from build123d import *
from build123d import SkipClean  # not in build123d's __all__

# Parameters (mm, degrees)
F0_W     = 71.95
F0_H     = 24.75
F1_DEPTH = 2
F2_DEPTH = 5


with BuildPart() as f1:
    # F0 (on Top) → F1 (new body)
    with BuildSketch(Plane.XY):
        with BuildLine():
            Line((34.5, 15), (-34.5, 15))
            ThreePointArc((-34.5, 15), (-36.6339745962, 12.1277186767), (-40, 13.3416876048))
            Line((-40, 13.3416876048), (-40, -14.8416876048))
            ThreePointArc((-40, -14.8416876048), (-37.4068848056, -13.5014454214), (-34.9019237886, -15))
            Line((-34.9019237886, -15), (34.9019237886, -15))
            ThreePointArc((34.9019237886, -15), (37.4068848056, -13.5014454214), (40, -14.8416876048))
            Line((40, -14.8416876048), (40, 13.3416876048))
            ThreePointArc((40, 13.3416876048), (36.6339745962, 12.1277186767), (34.5, 15))
        make_face()
        Rectangle(F0_W, F0_H, mode=Mode.SUBTRACT)
        with BuildLine():
            Line((-34.5, 15), (-36, 15))
            ThreePointArc((-36, 15), (-37.5, 13.5), (-39, 15))
            Line((-39, 15), (-40, 15))
            Line((-40, 15), (-40, 13.3416876048))
            ThreePointArc((-40, 13.3416876048), (-36.6339745962, 12.1277186767), (-34.5, 15))
        make_face()
        with BuildLine():
            Line((36, 15), (34.5, 15))
            ThreePointArc((34.5, 15), (36.6339745962, 12.1277186767), (40, 13.3416876048))
            Line((40, 13.3416876048), (40, 15))
            Line((40, 15), (39, 15))
            ThreePointArc((39, 15), (37.5, 13.5), (36, 15))
        make_face()
        with BuildLine():
            Line((40, -15), (40, -14.8416876048))
            ThreePointArc((40, -14.8416876048), (37.4068848056, -13.5014454214), (34.9019237886, -15))
            Line((34.9019237886, -15), (37.5, -15))
            Line((37.5, -15), (40, -15))
        make_face()
        with BuildLine():
            ThreePointArc((-34.9019237886, -15), (-37.4068848056, -13.5014454214), (-40, -14.8416876048))
            Line((-40, -14.8416876048), (-40, -15))
            Line((-40, -15), (-37.5, -15))
            Line((-37.5, -15), (-34.9019237886, -15))
        make_face()
    extrude(amount=F1_DEPTH)

    # F0 (on Top) → F2 (join)
    with BuildSketch(Plane.XY):
        with BuildLine():
            Line((-34.5, 15), (-36, 15))
            ThreePointArc((-36, 15), (-37.5, 13.5), (-39, 15))
            Line((-39, 15), (-40, 15))
            Line((-40, 15), (-40, 13.3416876048))
            ThreePointArc((-40, 13.3416876048), (-36.6339745962, 12.1277186767), (-34.5, 15))
        make_face()
        with BuildLine():
            ThreePointArc((-39, 15), (-37.5, 16.5), (-36, 15))
            Line((-36, 15), (-34.5, 15))
            ThreePointArc((-34.5, 15), (-38.3660254038, 17.8722813233), (-40, 13.3416876048))
            Line((-40, 13.3416876048), (-40, 15))
            Line((-40, 15), (-39, 15))
        make_face()
        with BuildLine():
            Line((-40, -15), (-40, -14.8416876048))
            ThreePointArc((-40, -14.8416876048), (-38.3660254038, -19.3722813233), (-34.5, -16.5))
            ThreePointArc((-34.5, -16.5), (-34.6022225211, -15.7235428647), (-34.9019237886, -15))
            Line((-34.9019237886, -15), (-37.5, -15))
            Line((-37.5, -15), (-40, -15))
        make_face()
        with BuildLine():
            ThreePointArc((-36, -16.5), (-38.5606601718, -17.5606601718), (-37.5, -15))
            ThreePointArc((-37.5, -15), (-36.4393398282, -15.4393398282), (-36, -16.5))
        make_face(mode=Mode.SUBTRACT)
        with BuildLine():
            ThreePointArc((-34.9019237886, -15), (-37.4068848056, -13.5014454214), (-40, -14.8416876048))
            Line((-40, -14.8416876048), (-40, -15))
            Line((-40, -15), (-37.5, -15))
            Line((-37.5, -15), (-34.9019237886, -15))
        make_face()
        with BuildLine():
            ThreePointArc((40.5, -16.5), (40.3722813233, -15.6339745962), (40, -14.8416876048))
            Line((40, -14.8416876048), (40, -15))
            Line((40, -15), (37.5, -15))
            Line((37.5, -15), (34.9019237886, -15))
            ThreePointArc((34.9019237886, -15), (36.7235428647, -19.3977774789), (40.5, -16.5))
        make_face()
        with BuildLine():
            ThreePointArc((39, -16.5), (36.4393398282, -17.5606601718), (37.5, -15))
            ThreePointArc((37.5, -15), (38.5606601718, -15.4393398282), (39, -16.5))
        make_face(mode=Mode.SUBTRACT)
        with BuildLine():
            Line((40, -15), (40, -14.8416876048))
            ThreePointArc((40, -14.8416876048), (37.4068848056, -13.5014454214), (34.9019237886, -15))
            Line((34.9019237886, -15), (37.5, -15))
            Line((37.5, -15), (40, -15))
        make_face()
        with BuildLine():
            ThreePointArc((40.5, 15), (37.5, 18), (34.5, 15))
            Line((34.5, 15), (36, 15))
            ThreePointArc((36, 15), (37.5, 16.5), (39, 15))
            Line((39, 15), (40, 15))
            Line((40, 15), (40, 13.3416876048))
            ThreePointArc((40, 13.3416876048), (40.3722813233, 14.1339745962), (40.5, 15))
        make_face()
        with BuildLine():
            Line((36, 15), (34.5, 15))
            ThreePointArc((34.5, 15), (36.6339745962, 12.1277186767), (40, 13.3416876048))
            Line((40, 13.3416876048), (40, 15))
            Line((40, 15), (39, 15))
            ThreePointArc((39, 15), (37.5, 13.5), (36, 15))
        make_face()
    with SkipClean():  # cleaning this boolean's faces spoils the solid; the shape is the same uncleaned
        extrude(amount=F2_DEPTH)


solid = f1.part
Verification items for the finished model (mm, model axes). A direction names the side the tool comes from. Coordinates: 2 decimals unless noted, no trailing zeros. Order: outer loops, then holes, each group sorted by start corner. A loop starts at its lowest first (then second) coordinate and runs counter-clockwise, first axis right, second up.
Item 1: Release check for a two-part mould opening along X. For faces 1 (the face through (-35.975, 0, 1)), 2 (the face through (-40, -1, 1)), 3 (the face through (0, -13, 2)), 4 (the face through (36, 14, 5)) record: +X half, -X half, draft (parallel to the pull), parting line (faces both ways), or undercut.
Filled in:
face 1: undercut
face 2: -X half
face 3: undercut
face 4: draft
Item 2: Material ranges on L1, parallel to Y at x = 37.5, z = 3.75; L2, parallel to Y at x = -37.5, z = 1.15; L3, parallel to X at y = -16.5, z = 2.35, recorded low to high.
Filled in:
L1: y = -19.5 to -18, -15 to -13.5, 12 to 13.5, 16.5 to 18
L2: y = -19.5 to -18, -15 to 13.5, 16.5 to 18
L3: x = -40.5 to -39, -36 to -34.5, 34.5 to 36, 39 to 40.5
Item 3: Depth check by flat-ended pin: pin 1 (2 mm diameter, centred on x = 23, z = 1, fed in from -Y); pin 2 (1.6 mm diameter, centred on y = -4, z = 0.5, fed in from -X); pin 3 (1.6 mm diameter, centred on x = 0.5, z = 1, fed in from +Y). Enter the tip coordinate at first touch or a pass-through.
Filled in:
pin 1: stops at y = -15
pin 2: stops at x = -40
pin 3: stops at y = 15
Item 4: Section check C-C, the plane x = 26.5. Enter the section's corners in (y, z) (3 decimals), then the cut area to 3 significant figures.
Filled in:
outline: (-15, 0) - (-12.375, 0) - (-12.375, 2) - (-15, 2) - close; (12.375, 0) - (15, 0) - (15, 2) - (12.375, 2) - close
area: 10.5 mm2
Item 5: Section check B-B, the plane z = 2.75. Enter the section's corners in (x, y).
Filled in:
outline: circle Ø6 at (-37.5, -16.5); circle Ø6 at (-37.5, 15); circle Ø6 at (37.5, -16.5); circle Ø6 at (37.5, 15); hole circle Ø3 at (-37.5, -16.5); hole circle Ø3 at (-37.5, 15); hole circle Ø3 at (37.5, -16.5); hole circle Ø3 at (37.5, 15)
Item 6: Section check A-A, the plane y = 5. Enter the section's corners in (x, z) (3 decimals), then the cut area to 3 significant figures.
Filled in:
outline: (-40, 0) - (-35.975, 0) - (-35.975, 2) - (-40, 2) - close; (35.975, 0) - (40, 0) - (40, 2) - (35.975, 2) - close
area: 16.1 mm2
Item 7: Access from +Z, -Z, +X, -X, +Y, -Y to the whole of each face (thin tool, end or side, straight path). Record for faces 5 (the face through (-1, -12.375, 1)), 6 (the face through (-3, -13, 0)), 7 (the face through (0, 15, 1)), 8 (the face through (40, -1, 1)).
Filled in:
face 5: +Z, -Z
face 6: -Z, +X, -X, +Y, -Y
face 7: +Z, -Z, +Y
face 8: +Z, -Z, +X
